Input: part model. Units: mm. Frame: model coordinates. Round coordinates to 2 decimals unless told otherwise and drop trailing zeros. Order: outer loops, then holes, each group sorted by start corner. A loop starts at its lowest first (then second) coordinate and runs counter-clockwise, first axis right, second up. Notation, with made-up numbers: (53, 45.5) - (104, 45.5) arc R20 cw to (104, 49.5) - close; hole circle Ø9 at (4.25, 73.25). An arc over 180 degrees is marked (long way). One line per item, written item: value. Start each with the question number.
from build123d import *

# Parameters (mm, degrees)
IZIM1_W                     = 294
IZIM1_H                     = 110
Y_KSEKLIK_EKSTR_ZYON1_DEPTH = 3
IZIM2_R                     = 50
KES_EKSTR_ZYON1_DEPTH       = 3


with BuildPart() as part:
    # Çizim1 → Yükseklik-Ekstrüzyon1 (new body)
    with BuildSketch(Plane(origin=(0, 0, 0), x_dir=(0, 0, -1), z_dir=(1, 0, 0))):
        with Locations((147, -55)):
            Rectangle(IZIM1_W, IZIM1_H)
    extrude(amount=Y_KSEKLIK_EKSTR_ZYON1_DEPTH)

    # Çizim2 → Kes-Ekstrüzyon1 (cut)
    with BuildSketch(Plane(origin=(3, 0, 0), x_dir=(0, 0, -1), z_dir=(1, 0, 0))):
        with Locations((214, -55)):
            Circle(IZIM2_R)
        with BuildLine():
            Line((35, -30), (35, -80))
            ThreePointArc((35, -80), (32.5, -82.5), (30, -80))
            Line((30, -80), (30, -30))
            ThreePointArc((30, -30), (32.5, -27.5), (35, -30))
        make_face()
        with BuildLine():
            Line((46.285714286, -30), (46.285714286, -80))
            ThreePointArc((46.285714286, -80), (48.785714286, -82.5), (51.285714286, -80))
            Line((51.285714286, -80), (51.285714286, -30))
            ThreePointArc((51.285714286, -30), (48.785714286, -27.5), (46.285714286, -30))
        make_face()
        with BuildLine():
            Line((62.571428571, -30), (62.571428571, -80))
            ThreePointArc((62.571428571, -80), (65.071428571, -82.5), (67.571428571, -80))
            Line((67.571428571, -80), (67.571428571, -30))
            ThreePointArc((67.571428571, -30), (65.071428571, -27.5), (62.571428571, -30))
        make_face()
        with BuildLine():
            Line((78.857142857, -30), (78.857142857, -80))
            ThreePointArc((78.857142857, -80), (81.357142857, -82.5), (83.857142857, -80))
            Line((83.857142857, -80), (83.857142857, -30))
            ThreePointArc((83.857142857, -30), (81.357142857, -27.5), (78.857142857, -30))
        make_face()
        with BuildLine():
            Line((95.142857143, -30), (95.142857143, -80))
            ThreePointArc((95.142857143, -80), (97.642857143, -82.5), (100.142857143, -80))
            Line((100.142857143, -80), (100.142857143, -30))
            ThreePointArc((100.142857143, -30), (97.642857143, -27.5), (95.142857143, -30))
        make_face()
        with BuildLine():
            Line((111.428571429, -30), (111.428571429, -80))
            ThreePointArc((111.428571429, -80), (113.928571429, -82.5), (116.428571429, -80))
            Line((116.428571429, -80), (116.428571429, -30))
            ThreePointArc((116.428571429, -30), (113.928571429, -27.5), (111.428571429, -30))
        make_face()
        with BuildLine():
            Line((127.714285714, -30), (127.714285714, -80))
            ThreePointArc((127.714285714, -80), (130.214285714, -82.5), (132.714285714, -80))
            Line((132.714285714, -80), (132.714285714, -30))
            ThreePointArc((132.714285714, -30), (130.214285714, -27.5), (127.714285714, -30))
        make_face()
        with BuildLine():
            Line((144, -30), (144, -80))
            ThreePointArc((144, -80), (146.5, -82.5), (149, -80))
            Line((149, -80), (149, -30))
            ThreePointArc((149, -30), (146.5, -27.5), (144, -30))
        make_face()
        with BuildLine():
            Line((48, -93), (62, -93))
            ThreePointArc((62, -93), (64.121320344, -93.878679656), (65, -96))
            Line((65, -96), (65, -100))
            ThreePointArc((65, -100), (64.121320344, -102.121320344), (62, -103))
            Line((62, -103), (48, -103))
            ThreePointArc((48, -103), (45.878679656, -102.121320344), (45, -100))
            Line((45, -100), (45, -96))
            ThreePointArc((45, -96), (45.878679656, -93.878679656), (48, -93))
        make_face()
    extrude(amount=-KES_EKSTR_ZYON1_DEPTH, mode=Mode.SUBTRACT)


solid = part.part
1. Section B-B (x = 0.65). State how many separate pieces and enclosed holes the cut face has, then the cut area to 3 significant figures.
2. Line query: line 1 (Y direction, x = 1.25, z = -213); line 2 (Y direction, x = 1.7, z = -54.5); line 3 (Y direction, x = 0.3, z = -50). Output: solid intervals per line, ascending. Write a range as from..to.
3. Section A-A (z = -214). Return the cut outline in (x, y).
4. Pull-direction query (Z, two-part tool) for faces 1 (the face through (0, -91, -145)), 2 (the face through (2, -85, -174)); classes: released by +Z, released by -Z, zero draft, split by the parting line, or undercut.
Solved:
1. separate pieces: 1
1. enclosed holes: 10
1. area: 22,100 mm²
2. line 1: y = -110..-104.99, -5.01..0
2. line 2: y = -110..-103, -93..0
2. line 3: y = -110..-103, -93..-82.19, -27.81..0
3. outline: (0, -110) - (3, -110) - (3, -105) - (0, -105) - close; (0, -5) - (3, -5) - (3, 0) - (0, 0) - close
4. face 1: zero draft
4. face 2: undercut
